Part model, mm, in its own coordinate system. Face numbers are marked on the shaded views. Coordinates: 2 decimals unless noted, no trailing zeros. Loops run counter-clockwise (first coordinate to the right, second up) from the corner with the lowest first, then second, coordinate; pieces in that order, holes last. Notation, with made-up numbers: M 74,-19.5 L 115,-19.5 A17 cw 115,9.5 Z; hole C -37,83 d3. An arc over 180 degrees is marked long. Answer as CSV lines item,"result". Start each with the question number.
from build123d import *

# Parameters (mm, degrees)
ESQUISSE1_W                = 650
ESQUISSE1_H                = 1400
ESQUISSE1_W_2              = 275
ESQUISSE1_H_2              = 550
ESQUISSE1_W_3              = 150
ESQUISSE1_W_4              = 500
ESQUISSE1_H_3              = 625
BOSS_EXTRU_1_DEPTH         = 63
R_P_TITION_LIN_AIRE1_COUNT = 2
R_P_TITION_LIN_AIRE1_PITCH = 300
ESQUISSE2_W                = 75
ESQUISSE2_H                = 75
ESQUISSE2_W_2              = 75.286628514
ESQUISSE2_W_3              = 74.984214748
BOSS_EXTRU_2_DEPTH         = 240
ESQUISSE15_R               = 10
ENL_V_MAT_EXTRU_4_DEPTH    = 1586.76218243


with BuildPart() as part:
    # Esquisse1 → Boss.-Extru.1 (new body)
    with BuildSketch(Plane.XY):
        with Locations((325, 700)):
            Rectangle(ESQUISSE1_W, ESQUISSE1_H)
        with Locations((212.5, 350)):
            Rectangle(ESQUISSE1_W_2, ESQUISSE1_H_2, mode=Mode.SUBTRACT)
        with Locations((500, 350)):
            Rectangle(ESQUISSE1_W_3, ESQUISSE1_H_2, mode=Mode.SUBTRACT)
        with Locations((325, 1012.5)):
            Rectangle(ESQUISSE1_W_4, ESQUISSE1_H_3, mode=Mode.SUBTRACT)
    extrude(amount=BOSS_EXTRU_1_DEPTH)


with BuildPart() as r_p_tition_lin_aire1_1:
    # R_p_tition lin_aire1: pattern copy
    add(part.part.moved(Location(Vector(0, 0, 1) * (1 * R_P_TITION_LIN_AIRE1_PITCH))))


with BuildPart() as part_1:
    add(part.part)

    add(r_p_tition_lin_aire1_1.part)  # Boss.-Extru.2 merges R_p_tition lin_aire1_1
    # Esquisse2 → Boss.-Extru.2 (add)
    with BuildSketch(Plane.XY.offset(63)):
        with Locations((37.5, 37.5)):
            Rectangle(ESQUISSE2_W, ESQUISSE2_H)
        with Locations((612.643314257, 37.5)):
            Rectangle(ESQUISSE2_W_2, ESQUISSE2_H)
        with Locations((612.492107374, 1362.5)):
            Rectangle(ESQUISSE2_W_3, ESQUISSE2_H)
        with Locations((37.5, 1362.5)):
            Rectangle(ESQUISSE2_W, ESQUISSE2_H)
    extrude(amount=BOSS_EXTRU_2_DEPTH)

    # Esquisse15 → Enl_v. mat.-Extru.4 (cut, through all)
    with BuildSketch(Plane(origin=(0, 0, 0), x_dir=(-1, 0, 0), z_dir=(0, 0, -1))):
        with Locations((-387.5, 662.5)):
            Circle(ESQUISSE15_R)
        with Locations((-387.5, 262.5)):
            Circle(ESQUISSE15_R)
    extrude(amount=-ENL_V_MAT_EXTRU_4_DEPTH, mode=Mode.SUBTRACT)


solid = part_1.part
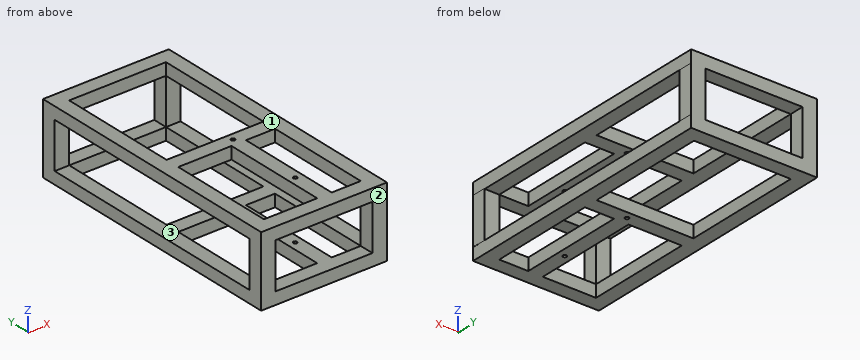
Q1. Slice it at A-A, the plane y = 747. Write the cut outline in (x, z), and give its area (3 significant figures).
Q2. Slice it at C-C, the plane x = 476.5. Write the cut outline in (y, z).
Q3. Slice it at B-B, the plane z = 268.5. Write the cut outline in (x, y), and give its area (3 significant figures).
Q4. Slice it at D-D, the plane y = 186. Write the cut outline in (x, z).
Q5. Two-plate mould, pull along Y, no slides. Class the marked faces 1, 2 and 3: +Y half, -Y half, draft (parallel to the pull), parting line (faces both ways), or undercut.
Q6. Wall check: L1, parallel to X at y = 167.5, z = 303; L2, parallel to Y at x = 387, z = 319; L3, parallel to X at y = 262, z = 329. Give the ranges that are in metal, low to high.
Solved:
1,outline,"M 0,0 L 75,0 L 75,63 L 0,63 Z; M 0,300 L 75,300 L 75,363 L 0,363 Z; M 575,0 L 650,0 L 650,63 L 575,63 Z; M 575,300 L 650,300 L 650,363 L 575,363 Z"
1,area,"18,900 mm2"
2,outline,"M 0,0 L 75,0 L 75,63 L 0,63 Z; M 0,300 L 75,300 L 75,363 L 0,363 Z; M 625,0 L 700,0 L 700,63 L 625,63 Z; M 625,300 L 700,300 L 700,363 L 625,363 Z; M 1325,0 L 1400,0 L 1400,63 L 1325,63 Z; M 1325,300 L 1400,300 L 1400,363 L 1325,363 Z"
3,outline,"M 0,0 L 75,0 L 75,75 L 0,75 Z; M 0,1325 L 75,1325 L 75,1400 L 0,1400 Z; M 575,0 L 650.29,0 L 650.29,75 L 575,75 Z; M 575,1325 L 649.98,1325 L 649.98,1400 L 575,1400 Z"
3,area,"22,500 mm2"
4,outline,"M 0,0 L 75,0 L 75,63 L 0,63 Z; M 0,300 L 75,300 L 75,363 L 0,363 Z; M 350,0 L 425,0 L 425,63 L 350,63 Z; M 350,300 L 425,300 L 425,363 L 350,363 Z; M 575,0 L 650,0 L 650,63 L 575,63 Z; M 575,300 L 650,300 L 650,363 L 575,363 Z"
5,face 1,"draft"
5,face 2,"-Y half"
5,face 3,"undercut"
6,L1,"x = 0 to 75, 350 to 425, 575 to 650"
6,L2,"y = 0 to 252.51, 272.49 to 652.51, 672.49 to 700, 1325 to 1400"
6,L3,"x = 0 to 75, 350 to 377.51, 397.49 to 425, 575 to 650"
